```python
from build123d import *

# Parameters (mm, degrees)
F0_R      = 9
F1_DEPTH  = 25
F2_W      = 12
F2_H      = 4
F3_DEPTH  = 15
F4_R      = 1.5
F5_DEPTH  = 12
F6_R      = 5.99999
F7_R      = 5.85
F8_DEPTH  = 17
F10_DEPTH = 8


# Not quite as in the source:
# - a fillet or chamfer is up to 0.001 mm smaller than in the source, because OpenCascade refuses the exact size


with BuildPart() as f1:
    # F0 (on Top) → F1 (new body)
    with BuildSketch(Plane.XY):
        Circle(F0_R)
    extrude(amount=F1_DEPTH)

    # F2 (on face) → F3 (join)
    with BuildSketch(Plane(origin=(0, 0, 0), x_dir=(1, 0, 0), z_dir=(0, 0, -1))):
        with Locations((0, -4)):
            Rectangle(F2_W, F2_H)
        with Locations((0, 4)):
            Rectangle(F2_W, F2_H)
    extrude(amount=F3_DEPTH)

    # F4 (on face) → F5 (cut, through all)
    with BuildSketch(Plane(origin=(0, 6, 0), x_dir=(-1, 0, 0), z_dir=(0, 1, 0))):
        with Locations((0, -7.464856375)):
            Circle(F4_R)
    extrude(amount=-F5_DEPTH, mode=Mode.SUBTRACT)

    # F6 (radius 6 in the source; OpenCascade refuses exactly that, so slightly less here)
    f6_edges = [f1.edges().sort_by_distance(p)[0] for p in [
        (-6, 4, -15),
        (-6, -4, -15),
        (6, -4, -15),
        (6, 4, -15),
    ]]
    fillet(f6_edges, radius=F6_R)

    # F7 (on face) → F8 (cut)
    with BuildSketch(Plane.XY.offset(25)):
        Circle(F7_R)
    extrude(amount=-F8_DEPTH, mode=Mode.SUBTRACT)

    # F9 (on face) → F10 (cut, through all)
    with BuildSketch(Plane(origin=(0, 0, 0), x_dir=(1, 0, 0), z_dir=(0, 0, -1))):
        with BuildLine():
            ThreePointArc((0, -2), (1.4142135624, -1.4142135624), (2, 0))
            ThreePointArc((2, 0), (1.4142135624, 1.4142135624), (0, 2))
            ThreePointArc((0, 2), (-2, 0), (0, -2))
        make_face()
    extrude(amount=-F10_DEPTH, mode=Mode.SUBTRACT)


solid = f1.part
```
Build history of the part. All positions in model axes, mm. A direction names the side the tool comes from. Round coordinates to 2 decimals unless told otherwise and drop trailing zeros. Write each loop counter-clockwise with the first axis right and the second up, starting at its lowest first coordinate (ties: lowest second). Pieces come first, ordered by that corner, then holes.
1) Band-saw the part on A-A, the plane z = -11. List the corners of the cut face in (x, y).
2) 3-axis set-ups, long thin cutter, end or side, ignore diameter. For faces 1 (the flat face through (-0.1, 6, -5.7)), 2 (the flat face through (6, -4, -4)), 3 (the flat face through (0, -3, 8)), 4 (the flat face through (-6, 4, -4)): which of +Z, -Z, +X, -X, +Y, -Y reach the whole face in a straight line?
3) Pin check, flat tips, straight feed: pin 1 (3 mm diameter, centred on y = -7, z = -4, fed in from +X); pin 2 (4 mm diameter, centred on y = 5.5, z = 17, fed in from +X); pin 3 (3 mm diameter, centred on y = -5.5, z = 14, fed in from -X). Stop position of each tip, or through.
4) Drill centre lines: probe 1 along Y at (x, z) = (0, 13.5); probe 2 along Y at (x, z) = (4.25, -10.5); probe 3 along Z at (x, y) = (0, 4.9). Where is each one in solid material? Low to high.
5) Band-saw the part on C-C, the plane x = 0.5. List the corners of the cut face in (y, z).
6) Mould opens along Z. For faces 5 (the cylindrical face through (0.33, -3.97, -8.93)), 6 (the flat face through (0, -6, 25)), 7 (the cylindrical face through (4.289, -4.028, -13.196)), 8 (the cylindrical face through (-1.27, -5.71, 16.62)) say: +Z half, -Z half, draft (parallel to the pull), parting line (faces both ways), or undercut.
7) Band-saw the part on D-D, the plane y = 0.75. List the corners of the cut face in (x, z).
Ans:
1. outline: (-5.66, -6) - (5.66, -6) - (5.66, -2) - (-5.66, -2) - close; (-5.66, 2) - (5.66, 2) - (5.66, 6) - (-5.66, 6) - close
2. face 1: -Z, +X, -X, +Y
2. face 2: -Z, +X, +Y, -Y
2. face 3: +Z
2. face 4: -Z, -X, +Y, -Y
3. pin 1: stops at x = 6
3. pin 2: stops at x = 8.29
3. pin 3: stops at x = -8.06
4. probe 1: y = -9 to -5.85, 5.85 to 9
4. probe 2: y = -6 to -2, 2 to 6
4. probe 3: z = -15 to -8.96, -5.96 to 8
5. outline: (-8.99, 0) - (-6, 0) - (-6, -6.05) - (-2, -6.05) - (-2, 0) - (-1.94, 0) - (-1.94, 8) - (-5.83, 8) - (-5.83, 25) - (-8.99, 25) - close; (-6, -14.98) - (-2, -14.98) - (-2, -8.88) - (-6, -8.88) - close; (1.94, 0) - (2, 0) - (2, -6.05) - (6, -6.05) - (6, 0) - (8.99, 0) - (8.99, 25) - (5.83, 25) - (5.83, 8) - (1.94, 8) - close; (2, -14.98) - (6, -14.98) - (6, -8.88) - (2, -8.88) - close
6. face 5: undercut
6. face 6: +Z half
6. face 7: -Z half
6. face 8: draft
7. outline: (-8.97, 0) - (-1.85, 0) - (-1.85, 8) - (-5.8, 8) - (-5.8, 25) - (-8.97, 25) - close; (1.85, 0) - (8.97, 0) - (8.97, 25) - (5.8, 25) - (5.8, 8) - (1.85, 8) - close
